```python
from build123d import *

# Parameters (mm, degrees)
SKETCH_1_W          = 22.95
SKETCH_1_H          = 19
SKETCH_1_W_2        = 75
SKETCH_1_W_3        = 98.4
EXTRUDE_7_DEPTH     = 2
SKETCH_4_R          = 15
CUT_EXTRUDE_1_DEPTH = 18
FILLET_1_R          = 3
FILLET_2_R          = 3
SKETCH_1_6_W        = 26.95
SKETCH_1_6_H        = 23
SKETCH_1_6_W_2      = 22.95
SKETCH_1_6_H_2      = 19
EXTRUDE_3_DEPTH     = 12
SKETCH_1_7_W        = 102.4
SKETCH_1_7_H        = 23
SKETCH_1_7_W_2      = 98.4
SKETCH_1_7_H_2      = 19
EXTRUDE_4_DEPTH     = 12
SKETCH_1_8_W        = 79
SKETCH_1_8_H        = 23
SKETCH_1_8_W_2      = 75
SKETCH_1_8_H_2      = 19
EXTRUDE_5_DEPTH     = 12
EXTRUDE_START       = 16
EXTRUDE_7_2_DEPTH   = 18
SKETCH_11_W         = 28.583123952
SKETCH_11_H         = 28.583123952
CUT_EXTRUDE_8_DEPTH = 10
EXTRUDE_START_2     = 2
SKETCH_13_W         = 14
SKETCH_13_H         = 14
EXTRUDE_8_DEPTH     = 2
SKETCH_15_W         = 14
SKETCH_15_H         = 14
EXTRUDE_9_DEPTH     = 2
EXTRUDE_START_3     = 8
EXTRUDE_12_DEPTH    = 8
CHAMFER_1_SIZE      = 1
CHAMFER_2_SIZE      = 1


with BuildPart() as part:
    # 草图1 → Extrude 7 (new body)
    with BuildSketch(Plane(origin=(0, 0, 0), x_dir=(1, 0, 0), z_dir=(0, 1, 0))):
        with BuildLine():
            Line((3, 0), (97, 0))
            ThreePointArc((97, 0), (99.121320344, 0.878679656), (100, 3))
            Line((100, 3), (100, 97))
            ThreePointArc((100, 97), (99.121320344, 99.121320344), (97, 100))
            Line((97, 100), (3, 100))
            ThreePointArc((3, 100), (0.878679656, 99.121320344), (0, 97))
            Line((0, 97), (0, 3))
            ThreePointArc((0, 3), (0.878679656, 0.878679656), (3, 0))
        make_face()
        with Locations((50, 77.8)):
            Rectangle(SKETCH_1_W, SKETCH_1_H, mode=Mode.SUBTRACT)
        with Locations((50, 10.3)):
            Rectangle(SKETCH_1_W_2, SKETCH_1_H, mode=Mode.SUBTRACT)
        with Locations((50, 53.8)):
            Rectangle(SKETCH_1_W_3, SKETCH_1_H, mode=Mode.SUBTRACT)
    extrude(amount=EXTRUDE_7_DEPTH)

    # 草图4 → 切除-拉伸1 (cut)
    with BuildSketch(Plane(origin=(0, 2, 0), x_dir=(1, 0, 0), z_dir=(0, 1, 0))):
        with Locations((10, 90)):
            Circle(SKETCH_4_R)
        with Locations((90, 90)):
            Circle(SKETCH_4_R)
    extrude(amount=-CUT_EXTRUDE_1_DEPTH, mode=Mode.SUBTRACT)

    # 圆角1
    fillet_1_edges = [part.edges().sort_by_distance(p)[0] for p in [
        (21.180339887, 1, -100),
        (0, 1, -78.819660113),
    ]]
    fillet(fillet_1_edges, radius=FILLET_1_R)

    # 圆角2
    fillet_2_edges = [part.edges().sort_by_distance(p)[0] for p in [
        (78.819660113, 1, -100),
        (100, 1, -78.819660113),
    ]]
    fillet(fillet_2_edges, radius=FILLET_2_R)

    # 草图1<6> → 拉伸-薄壁3 (add)
    with BuildSketch(Plane(origin=(0, 0, 0), x_dir=(1, 0, 0), z_dir=(0, 1, 0))):
        with Locations((50, 77.8)):
            Rectangle(SKETCH_1_6_W, SKETCH_1_6_H)
        with Locations((50, 77.8)):
            Rectangle(SKETCH_1_6_W_2, SKETCH_1_6_H_2, mode=Mode.SUBTRACT)
    extrude(amount=EXTRUDE_3_DEPTH)

    # 草图1<7> → 拉伸-薄壁4 (add)
    with BuildSketch(Plane(origin=(0, 0, 0), x_dir=(1, 0, 0), z_dir=(0, 1, 0))):
        with Locations((50, 53.8)):
            Rectangle(SKETCH_1_7_W, SKETCH_1_7_H)
        with Locations((50, 53.8)):
            Rectangle(SKETCH_1_7_W_2, SKETCH_1_7_H_2, mode=Mode.SUBTRACT)
    extrude(amount=EXTRUDE_4_DEPTH)

    # 草图1<8> → 拉伸-薄壁5 (add)
    with BuildSketch(Plane(origin=(0, 0, 0), x_dir=(1, 0, 0), z_dir=(0, 1, 0))):
        with Locations((50, 10.3)):
            Rectangle(SKETCH_1_8_W, SKETCH_1_8_H)
        with Locations((50, 10.3)):
            Rectangle(SKETCH_1_8_W_2, SKETCH_1_8_H_2, mode=Mode.SUBTRACT)
    extrude(amount=EXTRUDE_5_DEPTH)

    # 草图10 → Extrude 7 2 (add)
    with BuildSketch(Plane(origin=(0, 2, 0), x_dir=(1, 0, 0), z_dir=(0, 1, 0)).offset(EXTRUDE_START)):
        with BuildLine():
            Line((-2, 3), (-2, 73.416876048))
            ThreePointArc((-2, 73.416876048), (0.236146008, 77.583542715), (4.944444444, 78.023299368))
            ThreePointArc((4.944444444, 78.023299368), (19.192388155, 80.807611845), (21.976700632, 95.055555556))
            ThreePointArc((21.976700632, 95.055555556), (22.416457285, 99.763853992), (26.583123952, 102))
            Line((26.583123952, 102), (73.416876048, 102))
            ThreePointArc((73.416876048, 102), (77.583542715, 99.763853992), (78.023299368, 95.055555556))
            ThreePointArc((78.023299368, 95.055555556), (80.807611845, 80.807611845), (95.055555556, 78.023299368))
            ThreePointArc((95.055555556, 78.023299368), (99.763853992, 77.583542715), (102, 73.416876048))
            Line((102, 73.416876048), (102, 3))
            ThreePointArc((102, 3), (100.535533906, -0.535533906), (97, -2))
            Line((97, -2), (3, -2))
            ThreePointArc((3, -2), (-0.535533906, -0.535533906), (-2, 3))
        make_face()
        with BuildLine():
            Line((0, 3), (0, 73.416876048))
            ThreePointArc((0, 73.416876048), (1.341687605, 75.916876048), (4.166666667, 76.18073004))
            ThreePointArc((4.166666667, 76.18073004), (20.606601718, 79.393398282), (23.81926996, 95.833333333))
            ThreePointArc((23.81926996, 95.833333333), (24.083123952, 98.658312395), (26.583123952, 100))
            Line((26.583123952, 100), (73.416876048, 100))
            ThreePointArc((73.416876048, 100), (75.916876048, 98.658312395), (76.18073004, 95.833333333))
            ThreePointArc((76.18073004, 95.833333333), (79.393398282, 79.393398282), (95.833333333, 76.18073004))
            ThreePointArc((95.833333333, 76.18073004), (98.658312395, 75.916876048), (100, 73.416876048))
            Line((100, 73.416876048), (100, 3))
            ThreePointArc((100, 3), (99.121320344, 0.878679656), (97, 0))
            Line((97, 0), (3, 0))
            ThreePointArc((3, 0), (0.878679656, 0.878679656), (0, 3))
        make_face(mode=Mode.SUBTRACT)
    extrude(amount=-EXTRUDE_7_2_DEPTH)

    # 草图11 → 切除-拉伸8 (cut)
    with BuildSketch(Plane(origin=(0, 18, 0), x_dir=(1, 0, 0), z_dir=(0, 1, 0))):
        with Locations((87.708438024, 87.708438024)):
            Rectangle(SKETCH_11_W, SKETCH_11_H)
        with Locations((12.291561976, 87.708438024)):
            Rectangle(SKETCH_11_W, SKETCH_11_H)
    extrude(amount=-CUT_EXTRUDE_8_DEPTH, mode=Mode.SUBTRACT)

    # 草图13 → 凸台-拉伸8 (add)
    with BuildSketch(Plane(origin=(0, 8, 0), x_dir=(1, 0, 0), z_dir=(0, 1, 0)).offset(EXTRUDE_START_2)):
        with BuildLine():
            Line((26.583123952, 102), (26.583123952, 100))
            ThreePointArc((26.583123952, 100), (24.083123952, 98.658312395), (23.81926996, 95.833333333))
            ThreePointArc((23.81926996, 95.833333333), (20.606601718, 79.393398282), (4.166666667, 76.18073004))
            ThreePointArc((4.166666667, 76.18073004), (1.341687605, 75.916876048), (0, 73.416876048))
            Line((0, 73.416876048), (-2, 73.416876048))
            Line((-2, 73.416876048), (-2, 97))
            ThreePointArc((-2, 97), (-0.535533906, 100.535533906), (3, 102))
            Line((3, 102), (26.583123952, 102))
        make_face()
        with Locations((10, 90)):
            Rectangle(SKETCH_13_W, SKETCH_13_H, mode=Mode.SUBTRACT)
    extrude(amount=-EXTRUDE_8_DEPTH)

    # 草图15 → 凸台-拉伸9 (add)
    with BuildSketch(Plane(origin=(0, 8, 0), x_dir=(1, 0, 0), z_dir=(0, 1, 0)).offset(EXTRUDE_START_2)):
        with BuildLine():
            Line((73.416876048, 102), (97, 102))
            ThreePointArc((97, 102), (100.535533906, 100.535533906), (102, 97))
            Line((102, 97), (102, 73.416876048))
            Line((102, 73.416876048), (100, 73.416876048))
            ThreePointArc((100, 73.416876048), (98.658312395, 75.916876048), (95.833333333, 76.18073004))
            ThreePointArc((95.833333333, 76.18073004), (79.393398282, 79.393398282), (76.18073004, 95.833333333))
            ThreePointArc((76.18073004, 95.833333333), (75.916876048, 98.658312395), (73.416876048, 100))
            Line((73.416876048, 100), (73.416876048, 102))
        make_face()
        with Locations((90, 90)):
            Rectangle(SKETCH_15_W, SKETCH_15_H, mode=Mode.SUBTRACT)
    extrude(amount=-EXTRUDE_9_DEPTH)

    # 草图18 → 凸台-拉伸12 (add)
    with BuildSketch(Plane(origin=(0, 10, 0), x_dir=(1, 0, 0), z_dir=(0, 1, 0)).offset(EXTRUDE_START_3)):
        with BuildLine():
            Line((0, 73.416876048), (-2, 73.416876048))
            Line((-2, 73.416876048), (-2, 97))
            ThreePointArc((-2, 97), (-0.535533906, 100.535533906), (3, 102))
            Line((3, 102), (26.583123952, 102))
            Line((26.583123952, 102), (26.583123952, 100))
            Line((26.583123952, 100), (3, 100))
            ThreePointArc((3, 100), (0.878679656, 99.121320344), (0, 97))
            Line((0, 97), (0, 73.416876048))
        make_face()
        with BuildLine():
            Line((73.416876048, 102), (73.416876048, 100))
            Line((73.416876048, 100), (97, 100))
            ThreePointArc((97, 100), (99.121320344, 99.121320344), (100, 97))
            Line((100, 97), (100, 73.416876048))
            Line((100, 73.416876048), (102, 73.416876048))
            Line((102, 73.416876048), (102, 97))
            ThreePointArc((102, 97), (100.535533906, 100.535533906), (97, 102))
            Line((97, 102), (73.416876048, 102))
        make_face()
    extrude(amount=-EXTRUDE_12_DEPTH)

    # 倒角1
    chamfer_1_edges = [part.edges().sort_by_distance(p)[0] for p in [
        (50, 0, 2),
        (-0.535533906, 0, 0.535533906),
        (-2, 0, -38.208438024),
        (0.236146008, 0, -77.583542715),
        (22.416457285, 0, -99.763853992),
        (50, 0, -102),
        (77.583542715, 0, -99.763853992),
        (99.763853992, 0, -77.583542715),
        (102, 0, -38.208438024),
        (100.535533906, 0, 0.535533906),
        (80.807611845, 0, -80.807611845),
        (19.192388155, 0, -80.807611845),
    ]]
    chamfer(chamfer_1_edges, length=CHAMFER_1_SIZE)

    # 倒角2
    chamfer_2_edges = [part.edges().sort_by_distance(p)[0] for p in [
        (50, 18, 2),
        (100.535533906, 18, 0.535533906),
        (102, 18, -50),
        (50, 18, -102),
        (-2, 18, -50),
        (-0.535533906, 18, 0.535533906),
        (100.535533906, 18, -100.535533906),
        (-0.535533906, 18, -100.535533906),
    ]]
    chamfer(chamfer_2_edges, length=CHAMFER_2_SIZE)


solid = part.part
```
CAD build for the part. Positions are in the model's coordinates, mm. A direction names the side the tool comes from. Coordinates: 2 decimals unless noted, no trailing zeros. Loops run counter-clockwise (first coordinate to the right, second up) from the corner with the lowest first, then second, coordinate; pieces in that order, holes last. Notation, with made-up numbers: (32.25, 79) - (82.25, 79) arc R27 ccw to (82.25, 114) - close; hole circle Ø10 at (7, 70.25). An arc over 180 degrees is marked (long way). Return JSON: item names as keys, results as strings.
1. Mould opens along X. For faces 1 (the flat face through (38.525, 6, -78)), 2 (the flat face through (-2, 9, -49)), 3 (the flat face through (51, 9, 2)) say: released by +X, released by -X, zero draft, split by the parting line, or undercut.
Result:
{"face 1": "undercut", "face 2": "released by -X", "face 3": "zero draft"}
2. Band-saw the part on C-C (y = 13.5). Give the cut face in (x, z), and give its area (3 significant figures).
Result:
{"outline": "(-2, -97) arc R5 ccw to (3, -102) - (97, -102) arc R5 ccw to (102, -97) - (102, -3) arc R5 ccw to (97, 2) - (3, 2) arc R5 ccw to (-2, -3) - close; hole (0, -97) arc R3 ccw to (3, -100) - (97, -100) arc R3 ccw to (100, -97) - (100, -3) arc R3 ccw to (97, 0) - (3, 0) arc R3 ccw to (0, -3) - close", "area": "802 mm2"}
3. Drop flat-ended pins along their axis: pin 1 (6.5 mm diameter, centred on x = 41.5, z = -7, fed in from +Y); pin 2 (21 mm diameter, centred on x = 70, z = -31, fed in from +Y); pin 3 (3 mm diameter, centred on y = 5, z = -80, fed in from -X). Give the stop position or say it passes through.
Result:
{"pin 1": "passes through", "pin 2": "stops at y = 12", "pin 3": "stops at x = 16.06"}
4. Band-saw the part on A-A (x = 71.5). Give the cut face in (y, z), and give its area (3 significant figures).
Result:
{"outline": "(0, -101) - (1, -102) - (17, -102) - (18, -101) - (18, -100) - (2, -100) - (2, -65.3) - (12, -65.3) - (12, -63.3) - (0, -63.3) - close; (0, -44.3) - (12, -44.3) - (12, -42.3) - (2, -42.3) - (2, -21.8) - (12, -21.8) - (12, -19.8) - (0, -19.8) - close; (0, -0.8) - (12, -0.8) - (12, 0) - (18, 0) - (18, 1) - (17, 2) - (1, 2) - (0, 1) - close", "area": "262 mm2"}
5. 3-axis set-ups, long thin cutter, end or side, ignore diameter. For faces 4 (the cylindrical face through (99.71, 4.55, -77.62)), 5 (the cylindrical face through (100, 13, -101)), 6 (the flat face through (50, 6, -87.3)), 7 (the cylindrical face through (80.66, 4.55, -80.96)), 8 (the flat face through (49, 7, -42.3)): which of +Z, -Z, +X, -X, +Y, -Y reach the whole face in a straight line?
Result:
{"face 4": "-Z, -Y", "face 5": "-Z, +X, +Y, -Y", "face 6": "+Y, -Y", "face 7": "-Y", "face 8": "+Y"}
6. Probe L1, parallel to Z at x = 63, y = 6.5; L2, parallel to X at y = 5, z = -20.5; L3, parallel to Z at x = 80, y = 10.75. List the from-to ranges inside material, lowest first. Write a range as from..to.
Result:
{"L1": "z = -102..-100, -89.3..-66.3, -65.3..-63.3, -44.3..-42.3, -21.8..-19.8, -0.8..2", "L2": "x = -2..0, 10.5..89.5, 100..102", "L3": "z = -102..-100, -65.3..-63.3, -44.3..-42.3, -21.8..-19.8, -0.8..2"}
7. Band-saw the part on B-B (x = 55). State how many separate pieces and enclosed holes the cut face has, and give its area (3 significant figures).
Result:
{"separate pieces": "4", "enclosed holes": "0", "area": "264 mm2"}
8. Band-saw the part on D-D (z = -37.5). Give the cut face in (x, y), and give its area (3 significant figures).
Result:
{"outline": "(-2, 1) - (-1, 0) - (101, 0) - (102, 1) - (102, 17) - (101, 18) - (100, 18) - (100, 2) - (0, 2) - (0, 18) - (-1, 18) - (-2, 17) - close", "area": "270 mm2"}
